Geometry check sheet. Reference: the model listing, model coordinates, mm. A direction names the side the tool comes from. Coordinates: 2 decimals unless noted, no trailing zeros. Write each loop counter-clockwise with the first axis right and the second up, starting at its lowest first coordinate (ties: lowest second). Pieces come first, ordered by that corner, then holes. Notation, with made-up numbers: M 85,52 L 143,52 A16 cw 143,67 Z; hole C 20.25,5.5 d11. An arc over 180 degrees is marked long. Put each result on its own line as item: value. Start each with the question number.
1) Cross-section at C-C on x = -4.75. Record the cut outline in (y, z).
2) Cross-section at A-A on y = 33. Record the cut outline in (x, z), plus the area to 3 significant figures.
3) Mould release check, pull along Z, two halves, no side actions. Record for faces 4 (the flat face through (-3.091, 9.392, 34.874)), 5 (the flat face through (-4, 48, -62.065)), 6 (the flat face through (-3, 19.05, 43)): released by +Z, released by -Z, zero draft, split by the parting line, or undercut.
4) Scan lines: line 1 along Z through (x, y) = (-2.5, 12.5); line 2 along Y through (x, z) = (-0.5, -4); line 3 along X through (y, z) = (30, -41). Record each from-to range of solid material in increasing order.
5) Cross-section at B-B on z = 54. Record the cut outline in (x, y), plus the area to 3 significant figures.
6) Set-up check for faces 1 (the flat face through (-7, 100.279, -5)), 2 (the flat face through (-3, 0, 57)), 3 (the flat face through (-3, 19.05, 14)): record each of +Z, -Z, +X, -X, +Y, -Y from which the full face is reachable in a straight line by a thin tool's end or side.
7) Gauge pin test, flat ends, axial feed: pin 1 (3 mm diameter, centred on x = -2, z = -9.5, fed in from +Y); pin 2 (10 mm diameter, centred on y = 44, z = -29, fed in from +X); pin 3 (1.8 mm diameter, centred on x = -4.5, z = 28.5, fed in from +Y); pin 4 (1 mm diameter, centred on y = 86.5, z = 32, fed in from +X). Record the tip position at first contact, or that the pin passes through.
8) Cross-section at D-D on y = 6.5. Record the cut outline in (x, z).
Autodesk Inventor part; units mm, degrees
ref_plane "YZ Plane" through (0, 0, 0) normal (1, 0, 0) x (0, 1, 0)
ref_plane "XZ Plane" through (0, 0, 0) normal (0, 1, 0) x (-1, 0, 0)
ref_plane "XY Plane" through (0, 0, 0) normal (0, 0, 1) x (1, 0, 0)
sketch "Sketch1" plane through (0, 0, 0) normal (0, 1, 0) x (-1, 0, 0)
  line L0 (7.366, 0.1452) -> (7.366, -23.8548)
  line L1 (7.366, -23.8548) -> (0, -23.8548)
  line L2 (6.096, 4.754) -> (6.096, -4.754)
  line L3 (0, 4.754) -> (0, 7.802)
  line L4 (6.096, 7.802) -> (6.096, 4.754)
  line L5 (0, -4.754) -> (0, -7.548)
  line L6 (6.096, -7.802) -> (6.096, -4.754)
  line L7 (6.096, 7.802) -> (0, 4.754)
  line L8 (6.096, -7.802) -> (0, -4.754)
  line L9 (0, -23.8548) -> (0, -4.754)
  line L10 (0, 4.754) -> (0, 23.821)
  line L11 (6.096, 20.773) -> (6.096, 23.821)
  line L12 (6.096, 20.773) -> (0, 23.821)
  line L13 (6.096, 36.377) -> (6.096, 33.329)
  line L14 (6.096, 36.377) -> (0, 33.329)
  line L15 (6.096, 33.329) -> (6.096, 23.821)
  line L16 (6.096, 49.348) -> (6.096, 52.396)
  line L17 (6.096, 49.348) -> (0, 52.396)
  line L18 (6.096, 64.952) -> (6.096, 61.904)
  line L19 (6.096, 64.952) -> (0, 61.904)
  line L20 (6.096, 61.904) -> (6.096, 52.396)
  line L21 (6.096, 77.923) -> (6.096, 80.971)
  line L22 (6.096, 77.923) -> (0, 80.971)
  line L23 (6.096, 93.527) -> (6.096, 90.479)
  line L24 (6.096, 93.527) -> (0, 90.479)
  line L25 (6.096, 90.479) -> (6.096, 80.971)
  line L26 (7.366, 0.1452) -> (7.366, 101.147)
  line L27 (7.366, 101.147) -> (0, 101.147)
  line L28 (0, 33.329) -> (0, 52.396)
  line L29 (0, 61.904) -> (0, 80.971)
  line L30 (0, 90.479) -> (0, 101.147)
  point P0 (0, 0)
  dimension "d0" = 7.366
  dimension "d1" = 24
  dimension "d8" = 9.508
  dimension "d9" = 4.754
  dimension "d10" = 3.048
  dimension "d11" = 3.048
  dimension "d12" = 6.096
  dimension "d17" = 28.575
  dimension "d23" = 7.62
  dimension "d24" = 16.0528
  dimension "d31" = 125.0018
extrude "MultipleTeeth" add sketch "Sketch1" along normal blind 19.05
sketch "Sketch2" plane through (0, 0, 0) normal (0, -1, 0) x (1, 0, 0)
  line L0 (0, 4.754) -> (-6.096, 7.802) construction
  line L1 (-6.096, 7.802) -> (-6.096, -7.802) construction
  line L2 (-6.096, -7.802) -> (0, -4.754) construction
  line L3 (0, 23.821) -> (0, 4.754)
  line L4 (0, 4.754) -> (-6.096, 7.802)
  line L5 (-6.096, -7.802) -> (0, -4.754)
  line L6 (-6.096, 7.802) -> (-6.096, -7.802)
  line L7 (-6.096, -7.802) -> (-6.096, 7.802)
  line L8 (0, -4.754) -> (-6.096, -7.802)
  line L9 (-7.366, -23.8548) -> (-7.366, 101.147)
  line L10 (-7.366, -59.508) -> (-7.366, -32.8548)
  line L11 (-7.366, -23.8548) -> (0, -23.8548)
  line L12 (-7.366, 101.147) -> (0, 101.147)
  line L13 (-7.366, -55.8503) -> (-7.366, -40.458) construction
  line L14 (0, -43.0234) -> (0, -59.508) construction
  line L15 (-6.096, -62.0648) -> (0, -62.0648) construction
  line L16 (0, -32.8548) -> (0, -37.6258)
  line L17 (0, -49.9828) -> (0, -62.0648)
  line L18 (0, -62.0648) -> (0, -59.508)
  line L19 (0, -32.8548) -> (-7.366, -32.8548) construction
  line L20 (0, -51.9048) -> (-7.366, -51.9048) construction
  line L21 (0, -42.3798) -> (-7.366, -42.3798) construction
  line L22 (-6.096, -7.802) -> (-6.096, -62.0648) construction
  line L23 (0, -37.6258) -> (-6.096, -34.5778)
  line L24 (-6.096, -50.1818) -> (-6.096, -34.5778)
  line L25 (0, -47.1338) -> (-6.096, -50.1818)
  line L26 (0, -4.754) -> (0, -23.8548)
  line L27 (0, -23.8548) -> (0, -32.8548)
  line L28 (-7.366, -32.8548) -> (-7.366, -23.8548)
  line L29 (0, -49.9828) -> (0, -47.1338)
  line L30 (0, -62.0648) -> (-7.366, -62.0648)
  line L31 (-7.366, -62.0648) -> (-7.366, -59.508)
  point P0 (0, 0)
  dimension "d25" = 125.0018
  dimension "d33" = 9
  dimension "d34" = 19.05
  dimension "d36" = 9.525
  dimension "d38" = 10.16
extrude "LongTooth" add sketch "Sketch2" against normal blind 100.2792
sketch "Sketch3" plane through (0, 19.05, 0) normal (0, 1, 0) x (1, 0, 0)
  line L0 (-6.096, -7.802) -> (-6.096, 7.802) construction
  line L1 (0, 23.8548) -> (-7.366, 23.8548)
  line L2 (-7.366, -101.147) -> (0, -101.147)
  line L3 (-7.366, 23.8548) -> (-6.096, 23.8548)
  line L4 (-6.096, 23.8548) -> (-6.096, -101.147)
  line L5 (-6.096, -101.147) -> (-7.366, -101.147)
  line L6 (-7.366, -101.147) -> (-7.366, 23.8548)
  point P0 (0, 0)
extrude "ThinPlate" add sketch "Sketch3" along normal up to surface (81.2292 mm away)
sketch "Sketch4" plane through (0, 0, 0) normal (0, -1, 0) x (1, 0, 0)
  line L0 (-6.096, 101.147) -> (0, 101.147)
  line L1 (-7.366, 101.147) -> (-7.366, -62.0648)
  line L2 (0, 101.147) -> (-7.366, 101.147)
  line L3 (-7.366, 101.147) -> (-7.366, -62.0648)
  line L4 (-7.366, -62.0648) -> (0, -62.0648)
  line L5 (0, -62.0648) -> (0, 101.147)
  point P0 (0, 0)
extrude "Extrusion4" add sketch "Sketch4" along normal blind 5.08
equation "\"d11\" = d10"
equation "\"d36\" = 0.5 * d34"
properties part number "Sliding test receiver copy"
Answer key:
1. outline: M -5.08,-62.06 L 100.28,-62.06 L 100.28,-49.51 L 0,-49.51 L 0,-35.25 L 100.28,-35.25 L 100.28,-23.85 L 19.05,-23.85 L 19.05,-7.13 L 0,-7.13 L 0,7.13 L 19.05,7.13 L 19.05,21.45 L 0,21.45 L 0,35.7 L 19.05,35.7 L 19.05,50.02 L 0,50.02 L 0,64.28 L 19.05,64.28 L 19.05,78.6 L 0,78.6 L 0,92.85 L 19.05,92.85 L 19.05,101.15 L -5.08,101.15 Z
2. outline: M -7.37,-62.06 L 0,-62.06 L 0,-47.13 L -6.1,-50.18 L -6.1,-34.58 L 0,-37.63 L 0,-23.85 L -6.1,-23.85 L -6.1,101.15 L -7.37,101.15 Z
2. area: 364 mm²
3. face 4: undercut
3. face 5: released by -Z
3. face 6: zero draft
4. line 1: z = -62.06 to -48.38, -36.38 to -6, 6 to 22.57, 34.58 to 51.15, 63.15 to 79.72, 91.73 to 101.15
4. line 2: y = -5.08 to 0
4. line 3: x = -7.37 to -6.1
5. outline: M -7.37,-5.08 L 0,-5.08 L 0,0 L -6.1,0 L -6.1,100.28 L -7.37,100.28 Z
5. area: 165 mm²
6. face 1: +Z, -Z, +X, -X, +Y
6. face 2: +Y
6. face 3: +Z, +X, +Y
7. pin 1: stops at y = 19.05
7. pin 2: stops at x = 0
7. pin 3: stops at y = 0
7. pin 4: stops at x = -6.1
8. outline: M -7.37,-62.06 L 0,-62.06 L 0,-47.13 L -6.1,-50.18 L -6.1,-34.58 L 0,-37.63 L 0,-4.75 L -6.1,-7.8 L -6.1,7.8 L 0,4.75 L 0,23.82 L -6.1,20.77 L -6.1,36.38 L 0,33.33 L 0,52.4 L -6.1,49.35 L -6.1,64.95 L 0,61.9 L 0,80.97 L -6.1,77.92 L -6.1,93.53 L 0,90.48 L 0,101.15 L -7.37,101.15 Z
